Autodesk Inventor part; units mm, degrees
ref_plane "YZ Plane" through (0, 0, 0) normal (1, 0, 0) x (0, 1, 0)
ref_plane "XZ Plane" through (0, 0, 0) normal (0, 1, 0) x (-1, 0, 0)
ref_plane "XY Plane" through (0, 0, 0) normal (0, 0, 1) x (1, 0, 0)
sketch "Sketch1" plane through (0, 0, 0) normal (0, 1, 0) x (-1, 0, 0)
  circle A0 centre (0, 0) radius 3
  dimension "d2" = 6
extrude "Extrusion1" add sketch "Sketch1" along normal blind 50
chamfer "Chamfer1" distance 0.8 angle 45 2 edges at (3, 50, 0) (3, 0, 0)
sketch "Sketch2" plane through (0, 50, 0) normal (0, 1, 0) x (1, 0, 0)
  circle A0 centre (0, 0) radius 1.1
  dimension "d8" = 2.2
extrude "Extrusion2" cut sketch "Sketch2" against normal blind 10
properties part number "bar"
Could you check a few things on this model? Use its own coordinates, in mm. Round coordinates to 2 decimals unless told otherwise and drop trailing zeros. Write each loop counter-clockwise with the first axis right and the second up, starting at its lowest first coordinate (ties: lowest second). Pieces come first, ordered by that corner, then holes.
(1) Thinking about a two-plate mould opening in X: for faces 1 (the face through (1.05, 45.07, -0.33)), 2 (the face through (0, 40, 0)), 3 (the face through (3, 25, 0)), 4 (the face through (0, 0, 0)), which applies, +X half, -X half, draft (parallel to the pull), parting line (faces both ways), or undercut?
Findings below:
face 1: undercut
face 2: undercut
face 3: parting line
face 4: draft
(2) Suppose I cut it at D-D on y = 12. Write out the boundary of the cut face in (x, z).
Findings below:
outline: circle Ø6 at (0, 0)
(3) If I drill on probe 1 along Z at (x, y) = (0, 43); probe 2 along Z at (x, y) = (0.2, 9.5); probe 3 along X at (y, z) = (25, -0.1), over which ranges is the centre line in solid material (lowest first)?
Findings below:
probe 1: z = -3 to -1.1, 1.1 to 3
probe 2: z = -2.99 to 2.99
probe 3: x = -3 to 3
(4) Suppose I cut it at B-B on z = 0. Write out the boundary of the cut face in (x, y), and give its area (3 significant figures).
Findings below:
outline: (-3, 0.8) - (-2.2, 0) - (2.2, 0) - (3, 0.8) - (3, 49.2) - (2.2, 50) - (1.1, 50) - (1.1, 40) - (-1.1, 40) - (-1.1, 50) - (-2.2, 50) - (-3, 49.2) - close
area: 277 mm2
(5) Suppose I cut it at A-A on x = 0. Write out the boundary of the cut face in (y, z).
Findings below:
outline: (0, -2.2) - (0.8, -3) - (49.2, -3) - (50, -2.2) - (50, -1.1) - (40, -1.1) - (40, 1.1) - (50, 1.1) - (50, 2.2) - (49.2, 3) - (0.8, 3) - (0, 2.2) - close
(6) For pin 1 (2.5 mm diameter, centred on x = -0.5, z = 0.5, fed in from +Y); pin 2 (2 mm diameter, centred on y = 7.5, z = 2, fed in from -X); pin 3 (2 mm diameter, centred on x = 2, y = 32.5, fed in from +Z), each with a flat end and sliding along its axis, tell me the tip position at first contact or that it passes through.
Findings below:
pin 1: stops at y = 50
pin 2: stops at x = -2.83
pin 3: stops at z = 2.83
(7) Suppose I cut it at C-C on y = 46. Write out the boundary of the cut face in (x, z), and give its area (3 significant figures).
Findings below:
outline: circle Ø6 at (0, 0); hole circle Ø2.2 at (0, 0)
area: 24.5 mm2
